```python
from build123d import *

# Parameters (mm, degrees)
SKETCH1_W               = 80
SKETCH1_H               = 115
BOSS_EXTRUDE1_DEPTH     = 4
CUT_EXTRUDE1_REACH      = 6
SKETCH2_R               = 2.25
SKETCH4_W               = 3
SKETCH4_H               = 6
BOSS_EXTRUDE3_DEPTH     = 6
SKETCH5_R               = 1.55
CUT_EXTRUDE2_DEPTH      = 1
CUT_EXTRUDE2_DEPTH_BACK = 116
FILLET1_R               = 2
CUT_EXTRUDE3_REACH      = 6


with BuildPart() as part:
    # Sketch1 → Boss-Extrude1 (new body)
    with BuildSketch(Plane(origin=(0, 0, 0), x_dir=(0, 1, 0), z_dir=(0, 0, 1))):
        Rectangle(SKETCH1_W, SKETCH1_H)
    extrude(amount=BOSS_EXTRUDE1_DEPTH)

    # Sketch2 → Cut-Extrude1 (cut, up to next)
    with BuildSketch(Plane.XY.offset(4), mode=Mode.PRIVATE) as cut_extrude1_sk1:
        with Locations((13.25, 7.75)):
            Circle(SKETCH2_R)
    cut_extrude1_tool1 = extrude(cut_extrude1_sk1.sketch, amount=-CUT_EXTRUDE1_REACH, mode=Mode.PRIVATE) & part.part
    add(cut_extrude1_tool1.solids().sort_by_distance((13.25, 7.75, 4))[0], mode=Mode.SUBTRACT)
    # Sketch2 → Cut-Extrude1 (cut, up to next)
    with BuildSketch(Plane.XY.offset(4), mode=Mode.PRIVATE) as cut_extrude1_sk2:
        with Locations((-13.25, 7.75)):
            Circle(SKETCH2_R)
    cut_extrude1_tool2 = extrude(cut_extrude1_sk2.sketch, amount=-CUT_EXTRUDE1_REACH, mode=Mode.PRIVATE) & part.part
    add(cut_extrude1_tool2.solids().sort_by_distance((-13.25, 7.75, 4))[0], mode=Mode.SUBTRACT)
    # Sketch2 → Cut-Extrude1 (cut, up to next)
    with BuildSketch(Plane.XY.offset(4), mode=Mode.PRIVATE) as cut_extrude1_sk3:
        with Locations((13.25, -7.75)):
            Circle(SKETCH2_R)
    cut_extrude1_tool3 = extrude(cut_extrude1_sk3.sketch, amount=-CUT_EXTRUDE1_REACH, mode=Mode.PRIVATE) & part.part
    add(cut_extrude1_tool3.solids().sort_by_distance((13.25, -7.75, 4))[0], mode=Mode.SUBTRACT)
    # Sketch2 → Cut-Extrude1 (cut, up to next)
    with BuildSketch(Plane.XY.offset(4), mode=Mode.PRIVATE) as cut_extrude1_sk4:
        with Locations((-13.25, -7.75)):
            Circle(SKETCH2_R)
    cut_extrude1_tool4 = extrude(cut_extrude1_sk4.sketch, amount=-CUT_EXTRUDE1_REACH, mode=Mode.PRIVATE) & part.part
    add(cut_extrude1_tool4.solids().sort_by_distance((-13.25, -7.75, 4))[0], mode=Mode.SUBTRACT)

    # Sketch4 → Boss-Extrude3 (add)
    with BuildSketch(Plane(origin=(0, 0, 0), x_dir=(1, 0, 0), z_dir=(0, 0, -1))):
        with Locations((-56, 33)):
            Rectangle(SKETCH4_W, SKETCH4_H)
        with Locations((56, 33)):
            Rectangle(SKETCH4_W, SKETCH4_H)
        with Locations((-56, -33)):
            Rectangle(SKETCH4_W, SKETCH4_H)
        with Locations((56, -33)):
            Rectangle(SKETCH4_W, SKETCH4_H)
    extrude(amount=BOSS_EXTRUDE3_DEPTH)

    # Sketch5 → Cut-Extrude2 (cut, two sides)
    with BuildSketch(Plane.YZ.offset(57.5)) as cut_extrude2_sk:
        with Locations((-33, -3)):
            Circle(SKETCH5_R)
        with Locations((33, -3)):
            Circle(SKETCH5_R)
    extrude(amount=CUT_EXTRUDE2_DEPTH, mode=Mode.SUBTRACT)
    extrude(cut_extrude2_sk.sketch, amount=-CUT_EXTRUDE2_DEPTH_BACK, mode=Mode.SUBTRACT)

    # Fillet1
    fillet1_edges = [part.edges().sort_by_distance(p)[0] for p in [
        (56, 30, 0),
        (56, 36, 0),
        (56, 30, -6),
        (56, 36, -6),
        (-56, 30, 0),
        (-56, 36, 0),
        (-56, 30, -6),
        (-56, 36, -6),
        (-56, -30, 0),
        (-56, -36, 0),
        (-56, -30, -6),
        (-56, -36, -6),
        (56, -36, 0),
        (56, -30, 0),
        (56, -36, -6),
        (56, -30, -6),
    ]]
    fillet(fillet1_edges, radius=FILLET1_R)

    # Sketch6 → Cut-Extrude3 (cut, up to next)
    with BuildSketch(Plane(origin=(0, 0, 0), x_dir=(1, 0, 0), z_dir=(0, 0, -1)), mode=Mode.PRIVATE) as cut_extrude3_sk1:
        with BuildLine():
            Line((-42.5, 5), (-27.5, 5))
            ThreePointArc((-27.5, 5), (-22.5, 0), (-27.5, -5))
            Line((-27.5, -5), (-42.5, -5))
            ThreePointArc((-42.5, -5), (-47.5, 0), (-42.5, 5))
        make_face()
    cut_extrude3_tool1 = extrude(cut_extrude3_sk1.sketch, amount=-CUT_EXTRUDE3_REACH, mode=Mode.PRIVATE) & part.part
    add(cut_extrude3_tool1.solids().sort_by_distance((-35, 0, 0))[0], mode=Mode.SUBTRACT)


solid = part.part
```
Design review of the part built by this model. Coordinates are the model's own, in mm. A direction names the side the tool comes from. Coordinates: 2 decimals unless noted, no trailing zeros. Order: outer loops, then holes, each group sorted by start corner. A loop starts at its lowest first (then second) coordinate and runs counter-clockwise, first axis right, second up. Notation, with made-up numbers: (-25, 74) -> (29, 74) arc R18 ccw to (29, 84) -> close; hole circle Ø4 at (-29, 7). An arc over 180 degrees is marked (long way). One line per item, written item: value. Start each with the question number.
Q1. For probe 1 along Y at (x, z) = (-13.25, 2.95); probe 2 along Z at (x, y) = (55.4, 33); probe 3 along X at (y, z) = (-35.5, -5), list the stretches that pass through material, from the lowest coordinate up.
Q2. Take a section at B-B, the plane y = -7.75. State the section outline as (x, z) points, then the cut area to 3 significant figures.
Q3. Take a section at C-C, the plane x = 39.5. State the section outline as (y, z) points.
Q4. Insertion check: pin 1 Ø2 at (x, z) = (56, -3) entering from -Y; pin 2 Ø5 at (y, z) = (-33, -3) entering from -X; pin 3 Ø1.6 at (x, z) = (55.5, -3) entering from +Y; pin 4 Ø2 at (x, z) = (-56, -2.5) entering from +Y. Each pin has a flat end and moves straight along its axis. Give the tip position at first contact, or say it passes through.
Q5. Take a section at D-D, the plane y = 24. State the section outline as (x, z) points.
Q6. Take a section at A-A, the plane x = 13.25. State the section outline as (y, z) points, then the cut area to 3 significant figures.
Q7. Tool access review of faces 4 (the flat face through (54.5, -34, -1.6)), 5 (the flat face through (-35, 5, 2)), 6 (the cylindrical face through (56.021, 34.478, -2.534)): name each direction out of +Z, -Z, +X, -X, +Y, -Y from which nothing blocks a thin tool from reaching the whole face with its end or side.
Q8. Mouldability with a two-part tool opening along Y and no side actions: class faces 1 (the flat face through (1, 40, 2)), 2 (the flat face through (57.5, -1, 1)), 3 (the cylindrical face through (-12.04, 9.647, 2.028)) as pulls with the +Y half, pulls with the -Y half, needs draft (parallel to the pull), parting line crosses it, or undercut.
Values follow:
1. probe 1: y = -40 to -10, -5.5 to 5.5, 10 to 40
1. probe 2: z = -6 to -4.55, -1.45 to 4
1. probe 3: x = -57.5 to -54.5, 54.5 to 57.5
2. outline: (-57.5, 0) -> (-15.5, 0) -> (-15.5, 4) -> (-57.5, 4) -> close; (-11, 0) -> (11, 0) -> (11, 4) -> (-11, 4) -> close; (15.5, 0) -> (57.5, 0) -> (57.5, 4) -> (15.5, 4) -> close
2. area: 424 mm2
3. outline: (-40, 0) -> (40, 0) -> (40, 4) -> (-40, 4) -> close
4. pin 1: stops at y = -36
4. pin 2: stops at x = -57.5
4. pin 3: stops at y = 36
4. pin 4: stops at y = 36.06
5. outline: (-57.5, 0) -> (57.5, 0) -> (57.5, 4) -> (-57.5, 4) -> close
6. outline: (-40, 0) -> (-10, 0) -> (-10, 4) -> (-40, 4) -> close; (-5.5, 0) -> (5.5, 0) -> (5.5, 4) -> (-5.5, 4) -> close; (10, 0) -> (40, 0) -> (40, 4) -> (10, 4) -> close
6. area: 284 mm2
7. face 4: -Z, +Y, -Y
7. face 5: +Z, -Z
7. face 6: +X, -X
8. face 1: pulls with the +Y half
8. face 2: needs draft
8. face 3: undercut
